from build123d import *

# Parameters (mm, degrees)
SKICA1_R                 = 1.6
P_IDAT_VYSUNUT_M1_DEPTH  = 28
SKICA5_W                 = 33
SKICA5_H                 = 28.9
ODEBRAT_VYSUNUT_M3_DEPTH = 22
SKICA7_W                 = 30
SKICA7_H                 = 10.3
ODEBRAT_VYSUNUT_M5_DEPTH = 29
SKICA6_W                 = 47.5
SKICA6_H                 = 26
ODEBRAT_VYSUNUT_M4_DEPTH = 15.75
SKICA8_W                 = 50
SKICA8_H                 = 16
ODEBRAT_VYSUNUT_M6_DEPTH = 22
ODEBRAT_VYSUNUT_M7_DEPTH = 2.5


with BuildPart() as part:
    # Skica1 → Přidat vysunutím1 (new body)
    with BuildSketch(Plane.XY):
        with BuildLine():
            Line((19.45, -3.3), (-19.45, -3.3))
            ThreePointArc((-19.45, -3.3), (-21.783452378, -2.333452378), (-22.75, 0))
            Line((-22.75, 0), (-22.75, 41.5))
            ThreePointArc((-22.75, 41.5), (-21.783452378, 43.833452378), (-19.45, 44.8))
            Line((-19.45, 44.8), (19.45, 44.8))
            ThreePointArc((19.45, 44.8), (21.783452378, 43.833452378), (22.75, 41.5))
            Line((22.75, 41.5), (22.75, 0))
            ThreePointArc((22.75, 0), (21.783452378, -2.333452378), (19.45, -3.3))
        make_face()
        with Locations((19.45, 0)):
            Circle(SKICA1_R, mode=Mode.SUBTRACT)
        with Locations((-19.45, 0)):
            Circle(SKICA1_R, mode=Mode.SUBTRACT)
        with Locations((19.45, 41.5)):
            Circle(SKICA1_R, mode=Mode.SUBTRACT)
        with Locations((-19.45, 41.5)):
            Circle(SKICA1_R, mode=Mode.SUBTRACT)
    extrude(amount=P_IDAT_VYSUNUT_M1_DEPTH)

    # Skica5 → Odebrat vysunutím3 (cut)
    with BuildSketch(Plane.XY):
        with Locations((0, 10.15)):
            Rectangle(SKICA5_W, SKICA5_H)
    extrude(amount=ODEBRAT_VYSUNUT_M3_DEPTH, mode=Mode.SUBTRACT)

    # Skica7 → Odebrat vysunutím5 (cut, through all)
    with BuildSketch(Plane.XY):
        with Locations((0, 40.65)):
            Rectangle(SKICA7_W, SKICA7_H)
    extrude(amount=ODEBRAT_VYSUNUT_M5_DEPTH, mode=Mode.SUBTRACT)

    # Skica6 → Odebrat vysunutím4 (cut)
    with BuildSketch(Plane.XY):
        with Locations((0, 23.5)):
            Rectangle(SKICA6_W, SKICA6_H)
    extrude(amount=ODEBRAT_VYSUNUT_M4_DEPTH, mode=Mode.SUBTRACT)

    # Skica8 → Odebrat vysunutím6 (cut)
    with BuildSketch(Plane.XY):
        with Locations((0, 2.5)):
            Rectangle(SKICA8_W, SKICA8_H)
    extrude(amount=ODEBRAT_VYSUNUT_M6_DEPTH, mode=Mode.SUBTRACT)

    # Skica9 → Odebrat vysunutím7 (cut)
    with BuildSketch(Plane.XY.offset(22)):
        Polygon((-19.45, -3.233161507), (-19.45, -4.03299561), (-23.966905363, -4.03299561), (-23.966905363, 1.616580754), (-22.25, 1.616580754), (-19.45, 3.233161507), (-16.65, 1.616580754), (-16.65, -1.616580754), align=None)
    odebrat_vysunut_m7 = extrude(amount=ODEBRAT_VYSUNUT_M7_DEPTH, mode=Mode.SUBTRACT)

    # Zrcadlit1: Odebrat vysunutím7 across plane
    add(odebrat_vysunut_m7.mirror(Plane(origin=(0, 0, 0), x_dir=(0, 0, 1), z_dir=(1, 0, 0))), mode=Mode.SUBTRACT)


solid = part.part
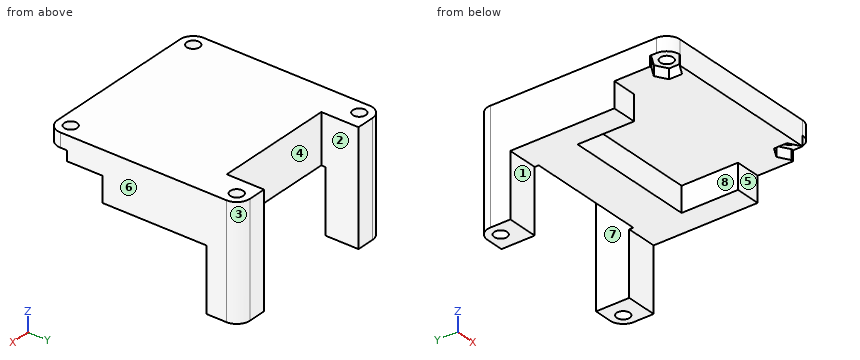
Here's how the part is built. I have some questions about the finished solid (model axes, mm). Face numbers are marked on the shaded views. A direction names the side the tool comes from. Round coordinates to 2 decimals unless told otherwise and drop trailing zeros. Order: outer loops, then holes, each group sorted by start corner. A loop starts at its lowest first (then second) coordinate and runs counter-clockwise, first axis right, second up. Notation, with made-up numbers: M 83,75.25 L 101,75.25 A9 ccw 101,83.25 Z; hole C 32.5,15.5 d5. An arc over 180 degrees is marked long. Return JSON: item names as keys, results as strings. Group by question number.
1. If we section it at C-C on y = 40.5: List the corners of the cut face in (x, z) for me, then the cut area to 3 significant figures.
2. I'm going to push flat-ended pins straight in: pin 1 Ø10 at (y, z) = (1.5, 17.5) entering from -X; pin 2 Ø3 at (x, z) = (-18.5, 19.5) entering from -Y; pin 3 Ø6 at (x, z) = (3, 19.5) entering from +Y; pin 4 Ø6 at (x, y) = (3, 15) entering from -Z. Where does each tip first touch, or does it pass through?
3. If we mould it in two halves opening along X, with no side actions, what happens to the marked faces 1, 2, 3 and 4? For each: pulls with the +X half, pulls with the -X half, needs draft (parallel to the pull), parting line crosses it, or undercut.
4. If we section it at A-A on z = 8: List the corners of the cut face in (x, y) for me, then the cut area to 3 significant figures.
5. Please list where these lines run through material, in increasing order: probe 1 along Y at (x, z) = (-19.45, 14); probe 2 along X at (y, z) = (40.5, 23); probe 3 along X at (y, z) = (39.5, 11.75).
6. If we section it at D-D on x = 12: List the corners of the cut face in (y, z) for me.
7. If we section it at B-B on z = 18: List the corners of the cut face in (x, y) for me.
8. On a 3-axis mill with a long thin cutter (end or side, diameter ignored), from which of +Z, -Z, +X, -X, +Y, -Y can I reach the whole of each face in a straight line? I mean the marked faces 5, 6, 7 and 8. Say none if no direction works.
Reply:
{
 "1": {"outline": "M -22.75,0 L -20.7,0 L -20.7,28 L -22.75,28 Z; M -18.2,0 L -15,0 L -15,28 L -18.2,28 Z; M 15,0 L 18.2,0 L 18.2,28 L 15,28 Z; M 20.7,0 L 22.75,0 L 22.75,28 L 20.7,28 Z", "area": "294 mm^2"},
 "2": {"pin 1": "x = -22.75", "pin 2": "y = 10.5", "pin 3": "y = 35.5", "pin 4": "z = 22"},
 "3": {"face 1": "needs draft", "face 2": "undercut", "face 3": "pulls with the +X half", "face 4": "undercut"},
 "4": {"outline": "M -22.75,36.5 L -15,36.5 L -15,44.8 L -19.45,44.8 A3.3 ccw -22.75,41.5 Z; M 15,36.5 L 22.75,36.5 L 22.75,41.5 A3.3 ccw 19.45,44.8 L 15,44.8 Z; hole C -19.45,41.5 d3.2; hole C 19.45,41.5 d3.2", "area": "108 mm^2"},
 "5": {"probe 1": "36.5 to 39.9, 43.1 to 44.8", "probe 2": "-22.75 to -20.7, -18.2 to -15, 15 to 18.2, 20.7 to 22.75", "probe 3": "-22.75 to -15, 15 to 22.75"},
 "6": {"outline": "M -3.3,22 L 24.6,22 L 24.6,15.75 L 35.5,15.75 L 35.5,28 L -3.3,28 Z"},
 "7": {"outline": "M -22.75,10.5 L -16.5,10.5 L -16.5,24.6 L 16.5,24.6 L 16.5,10.5 L 22.75,10.5 L 22.75,41.5 A3.3 ccw 19.45,44.8 L 15,44.8 L 15,35.5 L -15,35.5 L -15,44.8 L -19.45,44.8 A3.3 ccw -22.75,41.5 Z; hole C -19.45,41.5 d3.2; hole C 19.45,41.5 d3.2"},
 "8": {"face 5": "-Z, +X, -X, -Y", "face 6": "+Z, -Z, +X, +Y, -Y", "face 7": "+Z, -Z, +Y", "face 8": "-Z, -Y"}
}
